Read the model definition and answer for the solid it produces. Units are mm, in the model's axes. A direction names the side the tool comes from. Round coordinates to 2 decimals unless told otherwise and drop trailing zeros. Write each loop counter-clockwise with the first axis right and the second up, starting at its lowest first coordinate (ties: lowest second). Pieces come first, ordered by that corner, then holes. Notation, with made-up numbers: (84.5, -28.75) -> (138.5, -28.75) arc R12 cw to (138.5, -15.75) -> close; hole circle Ø11 at (2, -12). An arc over 180 degrees is marked (long way). Return JSON: item names as keys, results as strings.
from build123d import *

# Parameters (mm, degrees)
ESQUISSE1_R             = 22.5
BOSS_EXTRU_1_DEPTH      = 101
ESQUISSE2_R             = 22.5
ESQUISSE2_R_2           = 5
ENL_V_MAT_EXTRU_1_DEPTH = 70
ENL_V_START             = -28
ESQUISSE3_R             = 22.5
ESQUISSE3_R_2           = 11.25
ENL_V_MAT_EXTRU_2_DEPTH = 28
CONG_1_R                = 6
ESQUISSE6_W             = 6.909858745
ESQUISSE6_H             = 23.056365404
ENL_V_MAT_EXTRU_3_DEPTH = 20
ESQUISSE7_R             = 4
ENL_V_MAT_EXTRU_4_DEPTH = 108.736948259


with BuildPart() as part:
    # Esquisse1 → Boss.-Extru.1 (new body)
    with BuildSketch(Plane.XY):
        Circle(ESQUISSE1_R)
    extrude(amount=BOSS_EXTRU_1_DEPTH)

    # Esquisse2 → Enlèv. mat.-Extru.1 (cut)
    with BuildSketch(Plane(origin=(0, 0, 0), x_dir=(-1, 0, 0), z_dir=(0, 0, -1))):
        Circle(ESQUISSE2_R)
        Circle(ESQUISSE2_R_2, mode=Mode.SUBTRACT)
    extrude(amount=-ENL_V_MAT_EXTRU_1_DEPTH, mode=Mode.SUBTRACT)

    # Esquisse3 → Enlèv. mat.-Extru.2 (cut)
    with BuildSketch(Plane.XY.offset(101).offset(ENL_V_START)):
        with Locations(Location((0, 0, 0), (0, 0, 180))):
            Circle(ESQUISSE3_R)
        Circle(ESQUISSE3_R_2, mode=Mode.SUBTRACT)
    extrude(amount=ENL_V_MAT_EXTRU_2_DEPTH, mode=Mode.SUBTRACT)

    # Congé1
    cong_1_edges = [part.edges().sort_by_distance(p)[0] for p in [
        (-11.25, 0, 101),
    ]]
    fillet(cong_1_edges, radius=CONG_1_R)

    # Esquisse6 → Enlèv. mat.-Extru.3 (cut)
    with BuildSketch(Plane.XY.offset(101)):
        with Locations((10.954929373, 0)):
            Rectangle(ESQUISSE6_W, ESQUISSE6_H)
        with Locations((-10.954929373, 0)):
            Rectangle(ESQUISSE6_W, ESQUISSE6_H)
    extrude(amount=-ENL_V_MAT_EXTRU_3_DEPTH, mode=Mode.SUBTRACT)

    # Esquisse7 → Enlèv. mat.-Extru.4 (cut, through all)
    with BuildSketch(Plane(origin=(7.5, 0, 0), x_dir=(0, 0, -1), z_dir=(1, 0, 0))):
        with Locations(Location((-91, 0, 0), (0, 0, 90))):
            Circle(ESQUISSE7_R)
    extrude(amount=-ENL_V_MAT_EXTRU_4_DEPTH, mode=Mode.SUBTRACT)


solid = part.part
Item 1: Section B-B (x = 13.5) is taken. Give the vertices of the cut face in (y, z).
Worked answers:
{"outline": "(-18, 70) -> (18, 70) -> (18, 73) -> (-18, 73) -> close"}
Item 2: Straight lines are drawn through the part: L1, parallel to Z at x = 0.25, y = 0; L2, parallel to X at y = -6, z = 89; L3, parallel to Z at x = -11, y = 0.5. For each, find the intervals that lie inside material, in ascending order. Write a range as [from, to].
Worked answers:
{"L1": "z = [0, 87], [95, 101]", "L2": "x = [-7.5, 7.5]", "L3": "z = [70, 81]"}
Item 3: Flat-ended cylindrical pins translate along their axes: pin 1 (5 mm diameter, centred on x = -4, z = 48.5, fed in from -Y); pin 2 (13.5 mm diameter, centred on y = 4, z = 93.5, fed in from -X); pin 3 (18.5 mm diameter, centred on y = 3.5, z = 88, fed in from +X). Find the tip coordinate at first contact, or state that the pin passes through.
Worked answers:
{"pin 1": "stops at y = -4.77", "pin 2": "stops at x = -7.5", "pin 3": "stops at x = 11.25"}
Item 4: For a pull along Y with two mould halves and no side action, classify faces 4 (the cylindrical face through (0.105, 1.846, 87.451)), 5 (the flat face through (-7.5, -0.1, 86.6)), 6 (the cylindrical face through (1.08, -4.88, 34.51)) as released by +Y, released by -Y, zero draft, split by the parting line, or undercut.
Worked answers:
{"face 4": "undercut", "face 5": "zero draft", "face 6": "split by the parting line"}
Item 5: A tool of negligible diameter and unlimited length cuts with its end or side. For faces 1 (the flat face through (-9, 0, 81)), 2 (the flat face through (7.5, -0.1, 86.6)), 3 (the flat face through (5.3, -10.3, 73)), from which of +Z, -Z, +X, -X, +Y, -Y can it reach the whole face along a straight path? Write none if from no direction.
Worked answers:
{"face 1": "+Z, -X, +Y, -Y", "face 2": "+Z, +X, +Y, -Y", "face 3": "+Z"}
Item 6: Section C-C (z = 58.5) is taken. Give the vertices of the cut face in (x, y), then the cut area to 3 significant figures.
Worked answers:
{"outline": "circle Ø10 at (0, 0)", "area": "78.5 mm2"}
Item 7: Section D-D (x = -19) is taken. Give the vertices of the cut face in (y, z), then the cut area to 3 significant figures.
Worked answers:
{"outline": "(-12.05, 70) -> (12.05, 70) -> (12.05, 73) -> (-12.05, 73) -> close", "area": "72.3 mm2"}
Item 8: Section A-A (z = 91) is taken. Give the vertices of the cut face in (x, y).
Worked answers:
{"outline": "(-7.5, -8.39) arc R11.25 ccw to (7.5, -8.39) -> (7.5, -4) -> (-7.5, -4) -> close; (-7.5, 4) -> (7.5, 4) -> (7.5, 8.39) arc R11.25 ccw to (-7.5, 8.39) -> close"}
